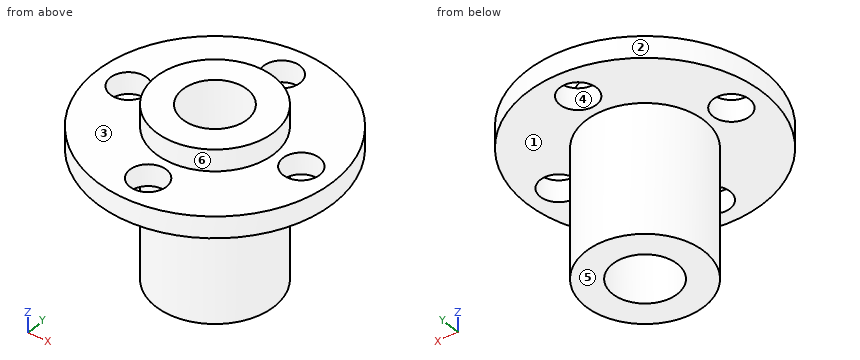
Solid Edge part; units mm, degrees
sketch "Sketch1" plane through (0, 0, 0) normal (0, -1, 0) x (1, 0, 0)
  line L0 (0, 4) -> (5.5, 4)
  line L1 (5.5, 4) -> (5.5, 2)
  line L2 (5.5, 2) -> (11, 2)
  line L3 (11, 2) -> (11, 0)
  line L4 (11, 0) -> (5.5, 0)
  line L5 (5.5, 0) -> (5.5, -12)
  line L6 (5.5, -12) -> (0, -12)
revolve "RevolvedProtrusion1" add sketch "Sketch1" angle 360 about axis through (0, 0, -12) along (0, 0, 1)
hole "Hole1" at (0, 0, 4) direction (0, 0, -1) diameter 6 end up to next
hole "Hole_2" at (-8, 0, 2) direction (0, 0, -1) diameter 3.4 end up to next
hole "Hole2" at (8, 0, 2) direction (0, 0, -1) diameter 3.4 end up to next
hole "Hole3" at (0, 8, 2) direction (0, 0, -1) diameter 3.4 end up to next
hole "Hole4" at (0, -8, 2) direction (0, 0, -1) diameter 3.4 end up to next
properties part number "A2.N2" material "Brass, yellow brass"
Geometry check sheet. Reference: the model listing, model coordinates, mm. Face numbers are marked on the shaded views. A direction names the side the tool comes from. Coordinates: 2 decimals unless noted, no trailing zeros. Order: outer loops, then holes, each group sorted by start corner. A loop starts at its lowest first (then second) coordinate and runs counter-clockwise, first axis right, second up. Notation, with made-up numbers: (-36, 69.5) - (14, 69.5) arc R12 ccw to (14, 79.5) - close; hole circle Ø6 at (30, 75). An arc over 180 degrees is marked (long way). One line per item, written item: value.
(1) Sectioned sample at D-D (y = -8). Enter the section's corners in (x, z).
Data:
outline: (-7.55, 0) - (-1.7, 0) - (-1.7, 2) - (-7.55, 2) - close; (1.7, 0) - (7.55, 0) - (7.55, 2) - (1.7, 2) - close
(2) Access from +Z, -Z, +X, -X, +Y, -Y to the whole of each face (thin tool, end or side, straight path). Record for the marked faces 1, 2 and 3.
Data:
face 1: -Z
face 2: +Z, -Z
face 3: +Z
(3) Thickness scan on probe 1 along Y at (x, z) = (0, -1.75); probe 2 along Z at (x, y) = (-1.5, -6.25); probe 3 along X at (y, z) = (2.5, -3.75). Record the ranges inside material, lowest first. Write a range as from..to.
Data:
probe 1: y = -5.5..-3, 3..5.5
probe 2: z = 0..2
probe 3: x = -4.9..-1.66, 1.66..4.9
(4) Release check for a two-part mould opening along Y. For the marked faces 4, 5 and 6 record: +Y half, -Y half, draft (parallel to the pull), parting line (faces both ways), or undercut.
Data:
face 4: undercut
face 5: draft
face 6: parting line
(5) Sectioned sample at A-A (y = 0). Enter the section's corners in (x, z), and give its area (3 significant figures).
Data:
outline: (-11, 0) - (-9.7, 0) - (-9.7, 2) - (-11, 2) - close; (-6.3, 0) - (-5.5, 0) - (-5.5, -12) - (-3, -12) - (-3, 4) - (-5.5, 4) - (-5.5, 2) - (-6.3, 2) - close; (3, -12) - (5.5, -12) - (5.5, 0) - (6.3, 0) - (6.3, 2) - (5.5, 2) - (5.5, 4) - (3, 4) - close; (9.7, 0) - (11, 0) - (11, 2) - (9.7, 2) - close
area: 88.4 mm^2
(6) Sectioned sample at C-C (x = 8.75). Enter the section's corners in (y, z).
Data:
outline: (-6.67, 0) - (-1.53, 0) - (-1.53, 2) - (-6.67, 2) - close; (1.53, 0) - (6.67, 0) - (6.67, 2) - (1.53, 2) - close
(7) Depth check by flat-ended pin: pin 1 Ø5 at (x, z) = (5, 2) entering from -Y; pin 2 Ø1 at (x, y) = (7, 0.5) entering from +Z; pin 3 Ø1 at (x, z) = (4.5, -8.5) entering from +Y; pin 4 Ø3 at (y, z) = (4.5, 2) entering from +X. Enter the tip coordinate at first touch or a pass-through.
Data:
pin 1: stops at y = -10.71
pin 2: passes through
pin 3: stops at y = 3.77
pin 4: stops at x = 10.58
